CAD build for the part. Positions are in the model's coordinates, mm. Face numbers are marked on the shaded views. A direction names the side the tool comes from. Give positions to 0.01 mm unless a question says otherwise; leave off trailing zeros. Loops run counter-clockwise (first coordinate to the right, second up) from the corner with the lowest first, then second, coordinate; pieces in that order, holes last. Notation, with made-up numbers: M -18,80.25 L 37,80.25 A18 ccw 37,113.25 Z; hole C 62,5 d11. An arc over 180 degrees is marked long. Answer as CSV lines item,"result".
```python
from build123d import *

# Parameters (mm, degrees)
F1_W     = 170
F1_H     = 100
F2_DEPTH = 25
F3_SIZE  = 18
F4_T     = -1.2
F5_R     = 3


with BuildPart() as f2:
    # F1 (on offset) → F2 (new body)
    with BuildSketch(Plane.XY.offset(25)):
        with Locations((0, -50)):
            Rectangle(F1_W, F1_H)
    extrude(amount=-F2_DEPTH)

    # F3
    f3_edges = [f2.edges().sort_by_distance(p)[0] for p in [
        (0, -100, 0),
        (85, -50, 0),
        (0, 0, 0),
        (-85, -50, 0),
    ]]
    chamfer(f3_edges, length=F3_SIZE)

    # F4
    f4_openings = [f2.faces().sort_by_distance(p)[0] for p in [
        (0, -50, 25),
    ]]
    offset(amount=F4_T, openings=f4_openings)

    # F5
    f5_edges = [f2.edges().sort_by_distance(p)[0] for p in [
        (0, -81.502944, 1.2),
        (66.502944, -50, 1.2),
        (0, -18.497056, 1.2),
        (-66.502944, -50, 1.2),
    ]]
    fillet(f5_edges, radius=F5_R)


solid = f2.part
```
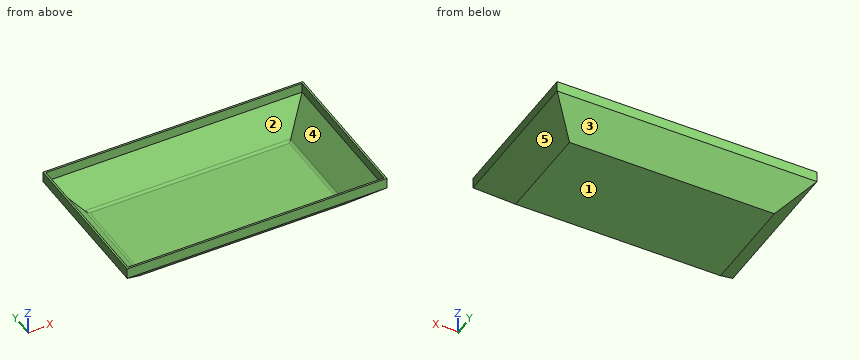
Q1. Mould opens along Y. For the marked faces 3, 4 and 5 say: released by +Y, released by -Y, zero draft, split by the parting line, or undercut.
Solution:
face 3,"released by +Y"
face 4,"undercut"
face 5,"zero draft"
Q2. Cut at B-B (z = 11.5). Write the cut outline in (x, y).
Solution:
outline,"M -78.5,-93.5 L 78.5,-93.5 L 78.5,-6.5 L -78.5,-6.5 Z; hole M -76.8,-91.8 L 76.8,-91.8 L 76.8,-8.2 L -76.8,-8.2 Z"
Q3. Pin check, flat tips, straight feed: P1, Ø1.5, axis at x = 40.5, y = -47.5, coming from the +Z side; P2, Ø5, axis at y = -89.5, z = 13.5, coming from the -X side; P3, Ø12, axis at x = 31, y = -22.5, coming from the +Z side. Stop position of each tip, or through.
Solution:
P1,"stops at z = 1.2"
P2,"stops at x = -83"
P3,"stops at z = 3.2"
Q4. Cut at C-C (y = -16). Write the cut outline in (x, z), and give its area (3 significant figures).
Solution:
outline,"M -85,18 L -69,2 L 69,2 L 85,18 L 85,25 L 83.8,25 L 83.8,18.5 L 69,3.7 L -69,3.7 L -83.8,18.5 L -83.8,25 L -85,25 Z"
area,"303 mm²"
Q5. Cut at A-A (x = 49.5). Write the cut outline in (y, z).
Solution:
outline,"M -100,18 L -82,0 L -18,0 L 0,18 L 0,25 L -1.2,25 L -1.2,18.5 L -17.62,2.08 A3 cw -19.74,1.2 L -80.26,1.2 A3 cw -82.38,2.08 L -98.8,18.5 L -98.8,25 L -100,25 Z"
Q6. Which spindle directions (+Z, -Z, +X, -X, +Y, -Y) get a long thin tool onto all of the face, cutting with end or side? Do the marked faces 1 and 2. Say none if no direction does.
Solution:
face 1,"-Z, +X, -X, +Y, -Y"
face 2,"+Z"
Q7. Cut at D-D (z = 23.25). Write the cut outline in (x, y).
Solution:
outline,"M -85,-100 L 85,-100 L 85,0 L -85,0 Z; hole M -83.8,-98.8 L 83.8,-98.8 L 83.8,-1.2 L -83.8,-1.2 Z"
Q8. Wall check: line 1 (X direction, y = -33, z = 22); line 2 (Y direction, x = -56.5, z = 22.5); line 3 (Z direction, x = -35, y = -53). Give the ranges that are in metal, low to high. Write a range as [from, to].
Solution:
line 1,"x = [-85, -83.8], [83.8, 85]"
line 2,"y = [-100, -98.8], [-1.2, 0]"
line 3,"z = [0, 1.2]"
